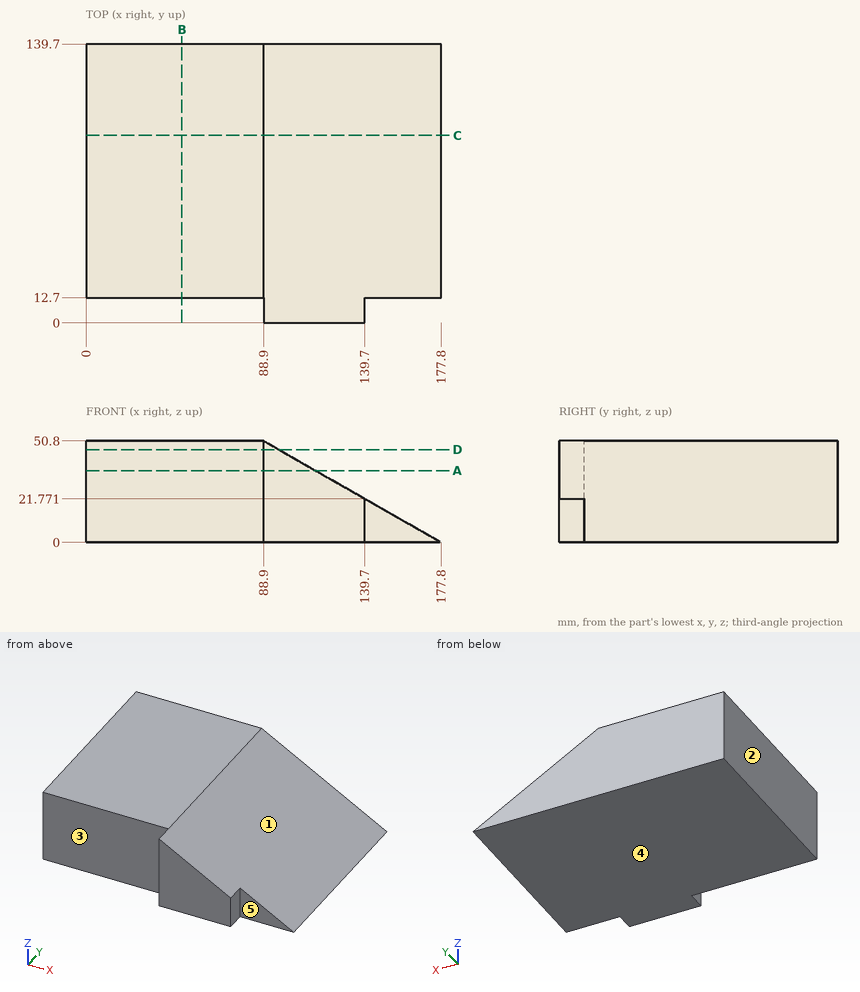
Answer from the drawing. Dimensions are ordinates in mm from the lowest x, y and z of the part. A direction names the side the tool comes from. Coordinates: 2 decimals unless noted, no trailing zeros. Write each loop counter-clockwise with the first axis right and the second up, starting at its lowest first coordinate (ties: lowest second). Pieces come first, ordered by that corner, then holes. Notation, with made-up numbers: M 54,-8.75 L 88,-8.75 A16 ccw 88,0.25 Z; hole C 35.25,78 d2. An arc over 180 degrees is marked long. Put each result on its own line as item: value. Start each with the question number.
1. A cutting plane is placed at D-D on z = 46.5. Write down the section's boundary in (x, y) (1 decimal), then the cut area to 3 significant figures.
2. Which of the six approach directions +Z, -Z, +X, -X, +Y, -Y give full straight-line access (tool end or side, diameter ignored) to the marked faces 4 and 5?
3. A cutting plane is placed at A-A on z = 36. Write down the section's boundary in (x, y), then the cut area to 3 significant figures.
4. A cutting plane is placed at C-C on y = 94. Write down the section's boundary in (x, z), then the cut area to 3 significant figures.
5. For a pull along X with two mould halves and no side action, classify the marked faces 1, 2 and 3 as pulls with the +X half, pulls with the -X half, needs draft (parallel to the pull), parting line crosses it, or undercut.
6. A cutting plane is placed at B-B on x = 48. Write down the section's boundary in (y, z).
7. Consider line 1 (Y direction, x = 51.5, z = 33.5); line 2 (X direction, y = 24, z = 43.5) (1 decimal); line 3 (X direction, y = 87.5, z = 39.5) (1 decimal). Determine where each line is inside the solid, lowest interval first. Write a range as from..to.
8. Flat-ended cylindrical pins translate along their axes: P1, Ø1.5, axis at x = 101, y = 47.5, coming from the +Z side (1 decimal); P2, Ø10, axis at y = 8.5, z = 19, coming from the -X side; P3, Ø10, axis at x = 155, y = 72, coming from the +Z side (1 decimal); P4, Ø12, axis at y = 53, z = 35.5, coming from the +X side (1 decimal). Find the tip coordinate at first contact, or state that the pin passes through.
Resolved:
1. outline: M 0,12.7 L 88.9,12.7 L 88.9,0 L 96.4,0 L 96.4,139.7 L 0,139.7 Z
1. area: 12,300 mm2
2. face 4: -Z, +X, -X, +Y, -Y
2. face 5: +Z, -Z, +X, -Y
3. outline: M 0,12.7 L 88.9,12.7 L 88.9,0 L 114.8,0 L 114.8,139.7 L 0,139.7 Z
3. area: 14,900 mm2
4. outline: M 0,0 L 177.8,0 L 88.9,50.8 L 0,50.8 Z
4. area: 6,770 mm2
5. face 1: pulls with the +X half
5. face 2: pulls with the -X half
5. face 3: needs draft
6. outline: M 12.7,0 L 139.7,0 L 139.7,50.8 L 12.7,50.8 Z
7. line 1: y = 12.7..139.7
7. line 2: x = 0..101.7
7. line 3: x = 0..108.7
8. P1: stops at z = 44.3
8. P2: stops at x = 0
8. P3: stops at z = 15.9
8. P4: stops at x = 126.2
